from build123d import *

# Parameters (mm, degrees)
F0_W     = 273.05
F0_H     = 114.3
F1_DEPTH = 19.05
F3_DEPTH = 25.4


with BuildPart() as f1:
    # F0 (on Front) → F1 (new body)
    with BuildSketch(Plane.XZ):
        with Locations((136.525, 57.15)):
            Rectangle(F0_W, F0_H)
    extrude(amount=F1_DEPTH)

    # F2 (on face) → F3 (cut)
    with BuildSketch(Plane.XZ.offset(19.05)):
        Polygon((21.852773, 12.687119), (0, 46.53658), (0, 0), (51.417489, 0), align=None)
        Polygon((273.05, 0), (273.05, 114.3), (226.663426, 66.674866), (165.820092, 25.969818), (133.684531, 7.116954), (92.12254, 0), align=None)
    extrude(amount=-F3_DEPTH, mode=Mode.SUBTRACT)


solid = f1.part
Can you work these out from the model? Positions are in its coordinate system, mm. Coordinates: 2 decimals unless noted, no trailing zeros. Order: outer loops, then holes, each group sorted by start corner. A loop starts at its lowest first (then second) coordinate and runs counter-clockwise, first axis right, second up. Notation, with made-up numbers: M 52,0 L 57,0 A19 cw 57,21 Z; hole C -27,89.5 d9. An arc over 180 degrees is marked long. Answer as CSV lines item,"result".
(1) I'm going to push flat-ended pins straight in: pin 1 (10 mm diameter, centred on y = -13.5, z = 44, fed in from +X); pin 2 (3 mm diameter, centred on x = 126, y = -17, fed in from -Z); pin 3 (1 mm diameter, centred on y = -9, z = 85, fed in from +X); pin 4 (8 mm diameter, centred on x = 238, z = 68.5, fed in from -Y). Where does each tip first touch, or does it pass through?
Geometry check:
pin 1,"x = 200.24"
pin 2,"z = 5.54"
pin 3,"x = 245"
pin 4,"through"
(2) Suppose I cut it at A-A on y = -15. Please give me the cut outline in (x, z), plus the area to 3 significant figures.
Geometry check:
outline,"M 0,46.54 L 21.85,12.69 L 51.42,0 L 92.12,0 L 133.68,7.12 L 165.82,25.97 L 226.66,66.67 L 273.05,114.3 L 0,114.3 Z"
area,"22,700 mm^2"
(3) Suppose I cut it at B-B on z = 56. Please give me the cut outline in (x, y), plus the area to 3 significant figures.
Geometry check:
outline,"M 0,-19.05 L 210.71,-19.05 L 210.71,0 L 0,0 Z"
area,"4,010 mm^2"
(4) Please list where these lines run through material, in increasing order: L1, parallel to X at y = -7.25, z = 60; L2, parallel to X at y = -0.75, z = 94; L3, parallel to Z at x = 163.5, y = -3.25.
Geometry check:
L1,"0 to 216.69"
L2,"0 to 253.28"
L3,"24.61 to 114.3"
(5) Suppose I cut it at C-C on x = 40.5. Please give me the cut outline in (y, z).
Geometry check:
outline,"M -19.05,4.69 L 0,4.69 L 0,114.3 L -19.05,114.3 Z"
